from build123d import *

# Parameters (mm, degrees)
CROQUIS1_W              = 9.25
CROQUIS1_H              = 114
CROQUIS1_H_2            = 10
CROQUIS1_R              = 2.5
SALIENTE_EXTRUIR1_DEPTH = 4.625
SALIENTE_EXTRUIR2_DEPTH = 12.5
CROQUIS1_4_W            = 9.25
CROQUIS1_4_H            = 10
CROQUIS1_4_R            = 2.5
CORTAR_EXTRUIR1_DEPTH   = 2.5
REDONDEO1_SIZE          = 4
REDONDEO2_SIZE          = 4.625
REDONDEO3_R             = 0.5
REDONDEO4_R             = 1


with BuildPart() as part:
    # Croquis1 → Saliente-Extruir1 (new, symmetric)
    # profile 1 of 2: a face of its own
    with BuildSketch(Plane.YZ):
        with Locations((0, 67)):
            Rectangle(CROQUIS1_W, CROQUIS1_H)
    # profile 2 of 2: a face of its own
    with BuildSketch(Plane.YZ):
        with Locations((0, 5)):
            Rectangle(CROQUIS1_W, CROQUIS1_H_2)
        with Locations(Location((0, 5, 0), (0, 0, 270))):
            Circle(CROQUIS1_R, mode=Mode.SUBTRACT)
    extrude(amount=SALIENTE_EXTRUIR1_DEPTH, both=True)

    # Croquis1<3> → Saliente-Extruir2 (add, symmetric)
    with BuildSketch(Plane.YZ):
        Polygon((4.625, 132), (-4.625, 132), (-4.625, 124), (4.625, 124), (8.375, 124), (8.375, 132), align=None)
    extrude(amount=SALIENTE_EXTRUIR2_DEPTH, both=True)

    # Croquis1<4> → Cortar-Extruir1 (cut, symmetric)
    with BuildSketch(Plane.YZ):
        with Locations((0, 5)):
            Rectangle(CROQUIS1_4_W, CROQUIS1_4_H)
        with Locations(Location((0, 5, 0), (0, 0, 270))):
            Circle(CROQUIS1_4_R, mode=Mode.SUBTRACT)
    extrude(amount=CORTAR_EXTRUIR1_DEPTH, both=True, mode=Mode.SUBTRACT)

    # Redondeo1
    # a fillet whose section is not a circle: 4 mm, written as the material it takes off along each edge
    with BuildSketch(Plane(origin=(14.625, -4.625, 0), x_dir=(0, 0, 1), z_dir=(-1, 0, 0)), Plane(origin=(14.625, 4.625, 0), x_dir=(0, -1, 0), z_dir=(-1, 0, 0))) as redondeo1_piece_1:
        with BuildLine():
            Bezier((REDONDEO1_SIZE, 0), (0, 0), (0, REDONDEO1_SIZE), weights=[1, 0.565685425, 1])
            Line((0, REDONDEO1_SIZE), (0, 0))
            Line((0, 0), (REDONDEO1_SIZE, 0))
        make_face()
    extrude(amount=22.125, mode=Mode.SUBTRACT)

    # Redondeo2
    # a fillet whose section is not a circle: 4.625 mm, written as the material it takes off along each edge
    with BuildSketch(Plane(origin=(-2.5, 4.625, 10), x_dir=(0, -1, 0), z_dir=(1, 0, 0)), Plane(origin=(-2.5, -4.625, 10), x_dir=(0, 0, 1), z_dir=(1, 0, 0))) as redondeo2_piece_1:
        with BuildLine():
            Bezier((REDONDEO2_SIZE, 0), (0, 0), (0, -REDONDEO2_SIZE), weights=[1, 0.817592216, 1])
            Line((0, -REDONDEO2_SIZE), (0, 0))
            Line((0, 0), (REDONDEO2_SIZE, 0))
        make_face()
    extrude(amount=5, mode=Mode.SUBTRACT)

    # Redondeo3
    redondeo3_edges = [part.edges().sort_by_distance(p)[0] for p in [
        (4.625, 4.625, 64),
        (4.625, 0, 0),
        (4.625, -4.625, 64),
        (4.625, 3.347604191, 1.277395809),
        (4.625, -3.347604191, 1.277395809),
        (-4.625, 0, 0),
        (-4.625, 3.347604191, 1.277395809),
        (-4.625, -3.347604191, 1.277395809),
        (-4.625, 4.625, 64),
        (-4.625, -4.625, 64),
    ]]
    fillet(redondeo3_edges, radius=REDONDEO3_R)

    # Redondeo4
    redondeo4_edges = [part.edges().sort_by_distance(p)[0] for p in [
        (12.5, 8.375, 128),
        (-12.5, -4.625, 128),
        (12.5, -4.625, 128),
        (-12.5, 8.375, 128),
    ]]
    fillet(redondeo4_edges, radius=REDONDEO4_R)


solid = part.part
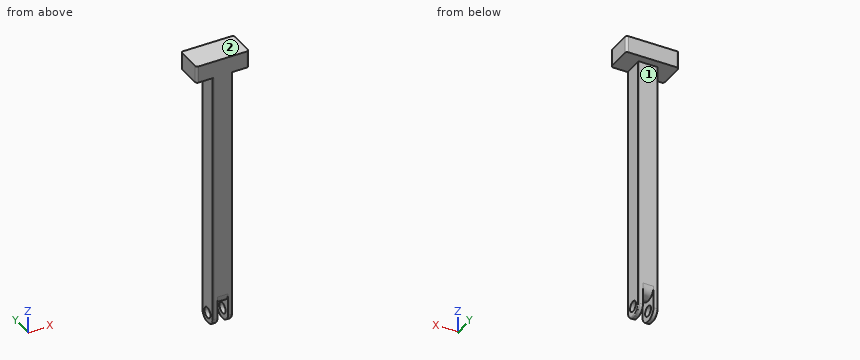
Design review of the part built by this model. Coordinates are the model's own, in mm. Face numbers are marked on the shaded views. A direction names the side the tool comes from. Give positions to 0.01 mm unless a question says otherwise; leave off trailing zeros. Loops run counter-clockwise (first coordinate to the right, second up) from the corner with the lowest first, then second, coordinate; pieces in that order, holes last. Notation, with made-up numbers: (4, -15) - (38, -15) arc R21 cw to (38, 15) - close; hole circle Ø1 at (-36, 12.5). An arc over 180 degrees is marked (long way). Use CSV: the item, a comma, the result in double quotes. Start each with the question number.
1. Wall thickness on L1, parallel to Y at x = 3.75, z = 5 (3 decimals); L2, parallel to X at y = -0.25, z = 20.5 (3 decimals); L3, parallel to Z at x = -6.5, y = -4: over which ranges is each line inside the solid? List them lowest first.
2. Add section A-A (z = 115.5). State the section outline as (x, y) points (3 decimals).
3. Insertion check: P1, Ø4, axis at y = 1, z = 68, coming from the +X side (3 decimals); P2, Ø4, axis at y = 1.5, z = 65.5, coming from the -X side (3 decimals); P3, Ø6.5, axis at x = 0, z = 90.5, coming from the +Y side (3 decimals). Each pin has a flat end and moves straight along its axis. Give the tip position at first contact, or say it passes through.
4. Machinability: for the marked faces 1 and 2, which of the approach directions +Z, -Z, +X, -X, +Y, -Y give a long, thin tool a straight path to every point of the face, cutting with its end or side? Answer none if there is none.
5. Add section B-B (x = -6.75). State the section outline as (y, z) points (3 decimals).
Results found:
1,L1,"y = -4.625 to -2.5, 2.5 to 4.625"
1,L2,"x = -4.625 to 4.625"
1,L3,"z = 124 to 132"
2,outline,"(-4.625, -4.125) arc R0.5 ccw to (-4.125, -4.625) - (4.125, -4.625) arc R0.5 ccw to (4.625, -4.125) - (4.625, 4.125) arc R0.5 ccw to (4.125, 4.625) - (-4.125, 4.625) arc R0.5 ccw to (-4.625, 4.125) - close"
3,P1,"stops at x = 4.625"
3,P2,"stops at x = -4.625"
3,P3,"stops at y = 4.625"
4,face 1,"-Z, +X, -X, +Y"
4,face 2,"+Z, +X, -X, +Y, -Y"
5,outline,"(-4.625, 124) - (8.375, 124) - (8.375, 132) - (-4.625, 132) - close"
